```python
from build123d import *

# Parameters (mm, degrees)
EXTRUDE_1_DEPTH          = 10
SKETCH_3_R               = 335.5
EXTRUDE_4_DEPTH          = 196
EXTRUDE_5_DEPTH          = 154.8
SHELL_START              = 10
SHELL_3_OUTLINE_R        = 330.5
SHELL_3_DEPTH            = 191
SHELL_3_2_DEPTH          = 149.8
CUT_EXTRUDE_1_DEPTH      = 154.8
SKETCH_8_R               = 80
EXTRUDE_7_DEPTH          = 61.8
SKETCH_9_R               = 80
EXTRUDE_8_DEPTH          = 123.6
SKETCH_10_R              = 75
CUT_EXTRUDE_2_DEPTH      = 185.4
SKETCH_11_R              = 10
CUT_EXTRUDE_4_DEPTH      = 1000
PATTERN_CIRCULAR_1_COUNT = 4


# Read off the part's stored shape, not the designer's step: 抽壳3
with BuildPart() as part:
    # 草图2 → 凸台-拉伸1 (new body)
    with BuildSketch(Plane(origin=(0, 0, 0), x_dir=(1, 0, 0), z_dir=(0, 1, 0))):
        with BuildLine():
            ThreePointArc((198.880672379, 401.826082595), (173.884394221, 413.257716136), (148.234596604, 423.136180053))
            Line((148.234596604, 423.136180053), (-143.504075774, 424.763819947))
            ThreePointArc((-143.504075774, 424.763819947), (-169.262499161, 415.172167754), (-194.384773816, 404.020150746))
            Line((-194.384773816, 404.020150746), (-401.826082595, 198.880672379))
            ThreePointArc((-401.826082595, 198.880672379), (-413.257716136, 173.884394221), (-423.136180053, 148.234596604))
            Line((-423.136180053, 148.234596604), (-424.763819947, -143.504075774))
            ThreePointArc((-424.763819947, -143.504075774), (-415.172167754, -169.262499161), (-404.020150746, -194.384773816))
            Line((-404.020150746, -194.384773816), (-198.880672379, -401.826082595))
            ThreePointArc((-198.880672379, -401.826082595), (-173.884394221, -413.257716136), (-148.234596604, -423.136180053))
            Line((-148.234596604, -423.136180053), (143.504075774, -424.763819947))
            ThreePointArc((143.504075774, -424.763819947), (169.262499161, -415.172167754), (194.384773816, -404.020150746))
            Line((194.384773816, -404.020150746), (401.826082595, -198.880672379))
            ThreePointArc((401.826082595, -198.880672379), (413.257716136, -173.884394221), (423.136180053, -148.234596604))
            Line((423.136180053, -148.234596604), (424.763819947, 143.504075774))
            ThreePointArc((424.763819947, 143.504075774), (415.172167754, 169.262499161), (404.020150746, 194.384773816))
            Line((404.020150746, 194.384773816), (198.880672379, 401.826082595))
        make_face()
    extrude(amount=EXTRUDE_1_DEPTH)

    # 草图7 → 切除-拉伸1 (cut)
    with BuildSketch(Plane.XZ.offset(-10)):
        with BuildLine():
            Line((354.410601365, 144.423875342), (292.048813878, 143.7280081))
            ThreePointArc((292.048813878, 143.7280081), (-325.4949343, -1.815969532), (293.634330198, -140.460421931))
            Line((293.634330198, -140.460421931), (356, -140.460421931))
            Line((356, -140.460421931), (356, 1.986160414))
            Line((356, 1.986160414), (354.410601365, 144.423875342))
        make_face()
    extrude(amount=CUT_EXTRUDE_1_DEPTH, mode=Mode.SUBTRACT)


with BuildPart() as body_2:
    # 草图3 → 凸台-拉伸4 (new body)
    with BuildSketch(Plane(origin=(0, 10, 0), x_dir=(1, 0, 0), z_dir=(0, 1, 0))):
        with Locations(Location((0, 0, 0), (0, 0, 270))):
            Circle(SKETCH_3_R)
    extrude(amount=EXTRUDE_4_DEPTH)


with BuildPart() as body_3:
    # 草图6 → 凸台-拉伸5 (new body)
    with BuildSketch(Plane(origin=(0, 10, 0), x_dir=(1, 0, 0), z_dir=(0, 1, 0))):
        with BuildLine():
            Line((366, -2.041951437), (335.494778671, -1.871759687))
            ThreePointArc((335.494778671, -1.871759687), (325.812555489, -80.040169201), (298.172341087, -153.796960343))
            Line((298.172341087, -153.796960343), (364.298400285, -154.534831406))
            Line((364.298400285, -154.534831406), (366, -2.041951437))
        make_face()
        with BuildLine():
            ThreePointArc((335.5, 0), (335.498694665, -0.935883485), (335.494778671, -1.871759687))
            Line((335.494778671, -1.871759687), (366, -2.041951437))
            Line((366, -2.041951437), (366, 150.460421931))
            Line((366, 150.460421931), (299.869824144, 150.460421931))
            ThreePointArc((299.869824144, 150.460421931), (326.470960424, 77.310814249), (335.5, 0))
        make_face()
    extrude(amount=EXTRUDE_5_DEPTH)


with BuildPart() as body_2_1:
    add(body_2.part)

    # Combine 1: union body 3
    add(body_3.part)

    # 抽壳3 outline → 抽壳3 (cut)
    with BuildSketch(Plane(origin=(0, 0, 0), x_dir=(1, 0, 0), z_dir=(0, 1, 0)).offset(SHELL_START)):
        Circle(SHELL_3_OUTLINE_R)
    extrude(amount=SHELL_3_DEPTH, mode=Mode.SUBTRACT)

    # Shell 3 2 outline → Shell 3 2 (cut)
    with BuildSketch(Plane(origin=(0, 0, 0), x_dir=(1, 0, 0), z_dir=(0, 1, 0)).offset(SHELL_START)):
        with BuildLine():
            ThreePointArc((296.76845461, 145.460421931), (330.494856485, -1.84386461), (295.126953902, -148.762666958))
            Line((295.126953902, -148.762666958), (359.354500825, -149.479353374))
            Line((359.354500825, -149.479353374), (361, -2.014055926))
            Line((361, -2.014055926), (361, 145.460421931))
            Line((361, 145.460421931), (296.76845461, 145.460421931))
        make_face()
    extrude(amount=SHELL_3_2_DEPTH, mode=Mode.SUBTRACT)

    # Combine 2: union part
    add(part.part)

    # 草图8 → 凸台-拉伸7 (add)
    with BuildSketch(Plane(origin=(0, 206, 0), x_dir=(1, 0, 0), z_dir=(0, 1, 0))):
        with Locations(Location((0, 0, 0), (0, 0, 270))):
            Circle(SKETCH_8_R)
    extrude(amount=EXTRUDE_7_DEPTH)

    # 草图9 → 凸台-拉伸8 (add)
    with BuildSketch(Plane(origin=(0, 201, 0), x_dir=(-1, 0, 0), z_dir=(0, -1, 0))):
        with Locations(Location((0, 0, 0), (0, 0, 270))):
            Circle(SKETCH_9_R)
    extrude(amount=EXTRUDE_8_DEPTH)

    # 草图10 → 切除-拉伸2 (cut)
    with BuildSketch(Plane.XZ.offset(-77.4)):
        with Locations(Location((0, 0, 0), (0, 0, 270))):
            Circle(SKETCH_10_R)
    extrude(amount=-CUT_EXTRUDE_2_DEPTH, mode=Mode.SUBTRACT)

    # 草图11 → 切除-拉伸4 (cut)
    with BuildSketch(Plane(origin=(0, 206, 0), x_dir=(1, 0, 0), z_dir=(0, 1, 0))):
        with Locations(Location((-229.340075244, 309.990589083, 0), (0, 0, 270))):
            Circle(SKETCH_11_R)
        with Locations(Location((-307.412348087, 232.784629383, 0), (0, 0, 270))):
            Circle(SKETCH_11_R)
    cut_extrude_4 = extrude(amount=-CUT_EXTRUDE_4_DEPTH, mode=Mode.SUBTRACT)

    # 阵列(圆周)1: 切除-拉伸4 ×4 about axis
    pattern_circular_1_axis = Axis((0, 0, 0), (0, 1, 0))
    for i in range(1, PATTERN_CIRCULAR_1_COUNT):
        add(cut_extrude_4.rotate(pattern_circular_1_axis, i * 360 / PATTERN_CIRCULAR_1_COUNT), mode=Mode.SUBTRACT)


solid = body_2_1.part
```
Check sheet for the modelled part. Datum: model origin and axes. Units: mm. A direction names the side the tool comes from. Give positions to 0.01 mm unless a question says otherwise; leave off trailing zeros. Order: outer loops, then holes, each group sorted by start corner. A loop starts at its lowest first (then second) coordinate and runs counter-clockwise, first axis right, second up. Notation, with made-up numbers: (45, -1.5) -> (92, -1.5) arc R28 cw to (92, 32.5) -> close; hole circle Ø7 at (34, -38.75). An arc over 180 degrees is marked (long way). Use CSV: the item, a comma, the result in double quotes. Start each with the question number.
1) Sectioned sample at C-C, the plane x = 0. Record the boundary of the cut face in (y, z), plus the area to 3 significant figures.
2) Material ranges on line 1 (X direction, y = 248.5, z = 6); line 2 (Z direction, x = 342.5, y = 137.5); line 3 (Z direction, x = 6, y = 40), recorded low to high. Write a range as from..to.
3) Go/stop test with flat-tipped pins: P1, Ø4, axis at y = 92, z = -228, coming from the -X side; P2, Ø6, axis at x = 83, y = 183, coming from the +Z side; P3, Ø18, axis at x = -307.41, z = -232.78, coming from the -Y side; P4, Ø3, axis at x = 332.5, y = 6.5, coming from the +Z side. Record where each tip stops, or that it passes through.
4) Sectioned sample at B-B, the plane z = -262. Record the boundary of the cut face in (x, y), plus the area to 3 significant figures.
5) Sectioned sample at D-D, the plane y = 231.5. Record the boundary of the cut face in (x, z).
6) Sectioned sample at A-A, the plane y = 48.5. Record the boundary of the cut face in (x, z).
7) Set-up check for faces 1 (the face through (-325.333, 5.07, 10.44)), 2 (the face through (329, 84, -145.46)), 3 (the face through (-78.1, 236.47, -17.34)), 4 (the face through (366, 86, -73)): record each of +Z, -Z, +X, -X, +Y, -Y from which the full face is reachable in a straight line by a thin tool's end or side.
8) Mould release check, pull along X, two halves, no side actions. Record for faces 5 (the face through (-70, 206, 70)), 6 (the face through (302.89, 4.93, -296.65)), 7 (the face through (342, 159.8, 0)): released by +X, released by -X, zero draft, split by the parting line, or undercut.
Recorded:
1,outline,"(0, -423.96) -> (10, -423.96) -> (10, -335.5) -> (206, -335.5) -> (206, -80) -> (267.8, -80) -> (267.8, 80) -> (206, 80) -> (206, 335.5) -> (10, 335.5) -> (10, 423.96) -> (0, 423.96) -> (0, 325.5) -> (10, 325.5) -> (10, 330.5) -> (201, 330.5) -> (201, 80) -> (77.4, 80) -> (77.4, 75) -> (262.8, 75) -> (262.8, -75) -> (77.4, -75) -> (77.4, -80) -> (201, -80) -> (201, -330.5) -> (10, -330.5) -> (10, -325.5) -> (0, -325.5) -> close"
1,area,"9,090 mm2"
2,line 1,"-79.77..-74.76, 74.76..79.77"
2,line 2,"-150.46..-145.46, 149.29..154.29"
2,line 3,"-335.45..-330.45, 330.45..335.45"
3,P1,"x = -247.96"
3,P2,"z = 325.82"
3,P3,"through"
3,P4,"z = 268.92"
4,outline,"(-338, 0) -> (-193.15, 0) -> (-193.15, 10) -> (-201.46, 10) -> (-201.46, 201) -> (201.46, 201) -> (201.46, 10) -> (193.15, 10) -> (193.15, 0) -> (337.16, 0) -> (337.16, 10) -> (209.56, 10) -> (209.56, 206) -> (-209.56, 206) -> (-209.56, 10) -> (-338, 10) -> close"
4,area,"8,080 mm2"
5,outline,"circle Ø160 at (0, 0); hole circle Ø150 at (0, 0)"
6,outline,"(298.17, 153.8) arc R335.5 ccw (long way) to (299.87, -150.46) -> (366, -150.46) -> (366, 2.04) -> (364.3, 154.53) -> close; hole (295.13, 148.76) arc R330.5 ccw (long way) to (296.77, -145.46) -> (361, -145.46) -> (361, 2.01) -> (359.35, 149.48) -> close"
7,face 1,"-Y"
7,face 2,"none"
7,face 3,"+Y"
7,face 4,"+Z, -Z, +X, +Y"
8,face 5,"zero draft"
8,face 6,"released by +X"
8,face 7,"undercut"
